Check sheet for the modelled part. Datum: model origin and axes. Units: mm. Round coordinates to 2 decimals unless told otherwise and drop trailing zeros. Loops run counter-clockwise (first coordinate to the right, second up) from the corner with the lowest first, then second, coordinate; pieces in that order, holes last. Notation, with made-up numbers: (-38.75, -23.75) - (-25.75, -23.75) arc R21 cw to (-25.75, -11.75) - close; hole circle Ø11 at (16.5, 47.25). An arc over 180 degrees is marked (long way). Return JSON: item names as keys, results as strings.
Autodesk Inventor part; units mm, degrees
ref_plane "YZ Plane" through (0, 0, 0) normal (1, 0, 0) x (0, 1, 0)
ref_plane "XZ Plane" through (0, 0, 0) normal (0, 1, 0) x (-1, 0, 0)
ref_plane "XY Plane" through (0, 0, 0) normal (0, 0, 1) x (1, 0, 0)
sketch "Skizze1" plane through (0, 0, 0) normal (0, 0, 1) x (1, 0, 0)
  circle A0 centre (0, 0) radius 2
  dimension "Durchmesser" = 4
extrude "Extrusion1" add sketch "Skizze1" along normal blind 55
chamfer "Fase1" distance 0.5 angle 45 1 edges at (-2, 0, 0) measured on face at (0.6473, -0.1595, 0)
chamfer "Fase2" distance 0.5 angle 45 1 edges at (-2, 0, 55) measured on face at (1.9935, -0.1609, 36.8333)
properties part number "ABI_Arretierstift"
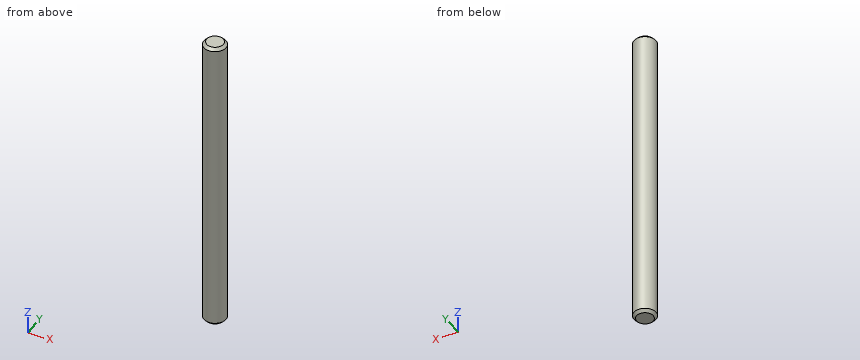
Q1. Depth check by flat-ended pin: P1, Ø1.5, axis at x = -1, y = -1, coming from the -Z side; P2, Ø1.5, axis at y = 1.5, z = 11.5, coming from the +X side. Enter the tip coordinate at first touch or a pass-through.
Answer key:
{"P1": "stops at z = 0", "P2": "stops at x = 1.85"}
Q2. Scan lines: probe 1 along Y at (x, z) = (-0.2, 40); probe 2 along X at (y, z) = (0.1, 6.5); probe 3 along X at (y, z) = (1.6, 32.5). Record each from-to range of solid material in increasing order. Write a range as [from, to].
Answer key:
{"probe 1": "y = [-1.99, 1.99]", "probe 2": "x = [-2, 2]", "probe 3": "x = [-1.2, 1.2]"}
Q3. Sectioned sample at A-A (z = 45.5). Enter the section's corners in (x, y), plus the area to 3 significant figures.
Answer key:
{"outline": "circle Ø4 at (0, 0)", "area": "12.6 mm²"}
